Geometry check sheet. Reference: the model listing, model coordinates, mm. Face numbers are marked on the shaded views. Coordinates: 2 decimals unless noted, no trailing zeros. Write each loop counter-clockwise with the first axis right and the second up, starting at its lowest first coordinate (ties: lowest second). Pieces come first, ordered by that corner, then holes. Notation, with made-up numbers: (76, -18) -> (94, -18) arc R23 cw to (94, 16) -> close; hole circle Ø5 at (21, -14). An arc over 180 degrees is marked (long way). One line per question, with ' | ' between items.
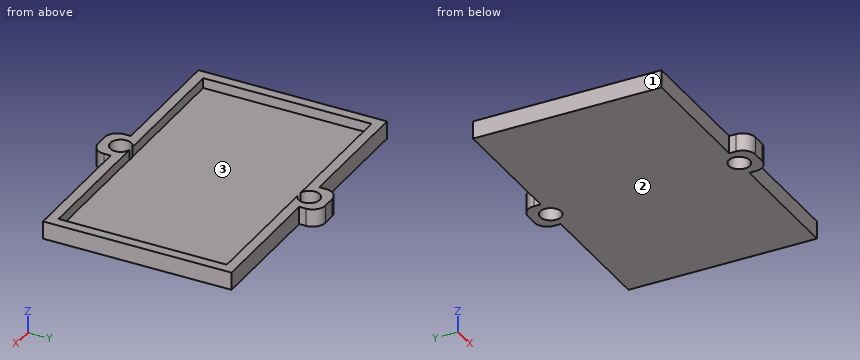
from build123d import *

# Parameters (mm, degrees)
F1_DEPTH = 2.4
F0_W     = 60
F0_H     = 35
F2_DEPTH = 1.8


# Not quite as in the source:
# - ends of sketch curves that miss each other by under 0.0002 mm in the source are joined


with BuildPart() as f1:
    # F0 (on Top) → F1 (new body)
    with BuildSketch(Plane.XY):
        Polygon((-32.7, -16.904), (-32.7, 22.896), (-4.8, 22.896), (-4.8, 25.2960002601), (-35.1000002601, 25.2960002601), (-35.1000002601, -19.3040002601), (-4.8, -19.3040002601), (-4.8, -16.904), align=None)
        Polygon((4.2, 25.2960002601), (4.2, 22.896), (32.1, 22.896), (32.1, -16.904), (4.2, -16.904), (4.2, -19.3040002601), (34.5000002601, -19.3040002601), (34.5000002601, 25.2960002601), align=None)
        with BuildLine():
            ThreePointArc((2.2, 25.296), (1.7, 23.796), (0.4, 22.896))
            Line((0.4, 22.896), (4.2, 22.896))
            Line((4.2, 22.896), (4.2, 25.2960002601))
            Line((4.2, 25.2960002601), (2.2, 25.296))
        make_face()
        with BuildLine():
            Line((-4.8, 25.2960002601), (-4.8, 22.896))
            Line((-4.8, 22.896), (-1, 22.896))
            ThreePointArc((-1, 22.896), (-2.300000078, 23.796000104), (-2.8, 25.2960002601))
            Line((-2.8, 25.2960002601), (-4.8, 25.2960002601))
        make_face()
        with BuildLine():
            Line((-4.8, 26.896), (-4.8, 25.2960002601))
            Line((-4.8, 25.2960002601), (-2.8, 25.2960002601))
            ThreePointArc((-2.8, 25.2960002601), (-0.2999998699, 27.796), (2.2, 25.296))
            Line((2.2, 25.296), (4.2, 25.2960002601))
            Line((4.2, 25.2960002601), (4.2, 26.896))
            ThreePointArc((4.2, 26.896), (3.3213203436, 29.0173203436), (1.2, 29.896))
            Line((1.2, 29.896), (-1.8, 29.896))
            ThreePointArc((-1.8, 29.896), (-3.9213203436, 29.0173203436), (-4.8, 26.896))
        make_face()
        with BuildLine():
            Line((-1, -16.904), (-4.8, -16.904))
            Line((-4.8, -16.904), (-4.8, -19.3040002601))
            Line((-4.8, -19.3040002601), (-4.8, -20.904))
            ThreePointArc((-4.8, -20.904), (-3.9213203436, -23.0253203436), (-1.8, -23.904))
            Line((-1.8, -23.904), (1.2, -23.904))
            ThreePointArc((1.2, -23.904), (3.3213203436, -23.0253203436), (4.2, -20.904))
            Line((4.2, -20.904), (4.2, -19.3040002601))
            Line((4.2, -19.3040002601), (4.2, -16.904))
            Line((4.2, -16.904), (0.4, -16.904))
            ThreePointArc((0.4, -16.904), (1.7, -17.804), (2.2, -19.304))
            ThreePointArc((2.2, -19.304), (-1.8, -21.304), (-1, -16.904))
        make_face()
    extrude(amount=F1_DEPTH)

    # F0 (on Top) → F2 (join)
    with BuildSketch(Plane.XY):
        Polygon((4.2, 25.2960002601), (4.2, 22.896), (32.1, 22.896), (32.1, -16.904), (4.2, -16.904), (4.2, -19.3040002601), (34.5000002601, -19.3040002601), (34.5000002601, 25.2960002601), align=None)
        with BuildLine():
            Line((-4.8, 22.896), (-32.7, 22.896))
            Line((-32.7, 22.896), (-32.7, -16.904))
            Line((-32.7, -16.904), (-4.8, -16.904))
            Line((-4.8, -16.904), (-1, -16.904))
            ThreePointArc((-1, -16.904), (-0.3, -16.804), (0.4, -16.904))
            Line((0.4, -16.904), (4.2, -16.904))
            Line((4.2, -16.904), (32.1, -16.904))
            Line((32.1, -16.904), (32.1, 22.896))
            Line((32.1, 22.896), (4.2, 22.896))
            Line((4.2, 22.896), (0.4, 22.896))
            ThreePointArc((0.4, 22.896), (-0.3, 22.796), (-1, 22.896))
            Line((-1, 22.896), (-4.8, 22.896))
        make_face()
        with Locations((-0.3, 2.996)):
            Rectangle(F0_W, F0_H, mode=Mode.SUBTRACT)
        with Locations((-0.3, 2.996)):
            Rectangle(F0_W, F0_H)
        Polygon((-32.7, -16.904), (-32.7, 22.896), (-4.8, 22.896), (-4.8, 25.2960002601), (-35.1000002601, 25.2960002601), (-35.1000002601, -19.3040002601), (-4.8, -19.3040002601), (-4.8, -16.904), align=None)
        with BuildLine():
            Line((-1, -16.904), (-4.8, -16.904))
            Line((-4.8, -16.904), (-4.8, -19.3040002601))
            Line((-4.8, -19.3040002601), (-4.8, -20.904))
            ThreePointArc((-4.8, -20.904), (-3.9213203436, -23.0253203436), (-1.8, -23.904))
            Line((-1.8, -23.904), (1.2, -23.904))
            ThreePointArc((1.2, -23.904), (3.3213203436, -23.0253203436), (4.2, -20.904))
            Line((4.2, -20.904), (4.2, -19.3040002601))
            Line((4.2, -19.3040002601), (4.2, -16.904))
            Line((4.2, -16.904), (0.4, -16.904))
            ThreePointArc((0.4, -16.904), (1.7, -17.804), (2.2, -19.304))
            ThreePointArc((2.2, -19.304), (-1.8, -21.304), (-1, -16.904))
        make_face()
        with BuildLine():
            Line((-4.8, 26.896), (-4.8, 25.2960002601))
            Line((-4.8, 25.2960002601), (-2.8, 25.2960002601))
            ThreePointArc((-2.8, 25.2960002601), (-0.2999998699, 27.796), (2.2, 25.296))
            Line((2.2, 25.296), (4.2, 25.2960002601))
            Line((4.2, 25.2960002601), (4.2, 26.896))
            ThreePointArc((4.2, 26.896), (3.3213203436, 29.0173203436), (1.2, 29.896))
            Line((1.2, 29.896), (-1.8, 29.896))
            ThreePointArc((-1.8, 29.896), (-3.9213203436, 29.0173203436), (-4.8, 26.896))
        make_face()
        with BuildLine():
            ThreePointArc((2.2, 25.296), (1.7, 23.796), (0.4, 22.896))
            Line((0.4, 22.896), (4.2, 22.896))
            Line((4.2, 22.896), (4.2, 25.2960002601))
            Line((4.2, 25.2960002601), (2.2, 25.296))
        make_face()
        with BuildLine():
            Line((-4.8, 25.2960002601), (-4.8, 22.896))
            Line((-4.8, 22.896), (-1, 22.896))
            ThreePointArc((-1, 22.896), (-2.300000078, 23.796000104), (-2.8, 25.2960002601))
            Line((-2.8, 25.2960002601), (-4.8, 25.2960002601))
        make_face()
    extrude(amount=-F2_DEPTH)


solid = f1.part
1. Material ranges on line 1 (Y direction, x = -0.3, z = -0.05); line 2 (Y direction, x = -0.3, z = 0.35); line 3 (X direction, y = -5.5, z = 0.35), recorded low to high. Write a range as from..to.
Worked answers:
line 1: -23.9..-21.8, -16.8..22.8, 27.8..29.9 | line 2: -23.9..-21.8, 27.8..29.9 | line 3: -35.1..-32.7, 32.1..34.5
2. Cross-section at A-A on z = -1.05. Record the boundary of the cut face in (x, y), and give its area (3 significant figures).
Worked answers:
outline: (-35.1, -19.3) -> (-4.8, -19.3) -> (-4.8, -20.9) arc R3 ccw to (-1.8, -23.9) -> (1.2, -23.9) arc R3 ccw to (4.2, -20.9) -> (4.2, -19.3) -> (34.5, -19.3) -> (34.5, 25.3) -> (4.2, 25.3) -> (4.2, 26.9) arc R3 ccw to (1.2, 29.9) -> (-1.8, 29.9) arc R3 ccw to (-4.8, 26.9) -> (-4.8, 25.3) -> (-35.1, 25.3) -> close; hole circle Ø5 at (-0.3, -19.3); hole circle Ø5 at (-0.3, 25.3) | area: 3,140 mm²
3. Cross-section at B-B on x = -28.5. Record the boundary of the cut face in (y, z).
Worked answers:
outline: (-19.3, -1.8) -> (25.3, -1.8) -> (25.3, 2.4) -> (22.9, 2.4) -> (22.9, 0) -> (-16.9, 0) -> (-16.9, 2.4) -> (-19.3, 2.4) -> close
4. Mould release check, pull along X, two halves, no side actions. Record for the marked faces 1, 2 and 3: released by +X, released by -X, zero draft, split by the parting line, or undercut.
Worked answers:
face 1: released by -X | face 2: zero draft | face 3: undercut
5. Cross-section at C-C on y = -3.5. Record the boundary of the cut face in (x, z), and give its area (3 significant figures).
Worked answers:
outline: (-35.1, -1.8) -> (34.5, -1.8) -> (34.5, 2.4) -> (32.1, 2.4) -> (32.1, 0) -> (-32.7, 0) -> (-32.7, 2.4) -> (-35.1, 2.4) -> close | area: 137 mm²
6. Go/stop test with flat-tipped pins: P1, Ø0.5, axis at y = 26.5, z = 1, coming from the +X side; P2, Ø1.3, axis at y = -20, z = -0.5, coming from the -X side; P3, Ø1, axis at x = 16.5, z = -0.5, coming from the +Y side; P4, Ø4.5, axis at x = -0.3, y = 25.296, coming from the +Z side. Record where each tip stops, or that it passes through.
Worked answers:
P1: x = 4.2 | P2: x = -4.8 | P3: y = 25.3 | P4: through
